Geometry check sheet. Reference: the model listing, model coordinates, mm. Face numbers are marked on the shaded views. A direction names the side the tool comes from. Give positions to 0.01 mm unless a question says otherwise; leave off trailing zeros. Write each loop counter-clockwise with the first axis right and the second up, starting at its lowest first coordinate (ties: lowest second). Pieces come first, ordered by that corner, then holes.
(1) Cross-section at A-A (z = -4). Record the boundary of the cut face in (x, y) (3 decimals).
(2) Mould release check, pull along X, two halves, no side actions. Record for the marked faces 6, 7 and 8: +X half, -X half, draft (parallel to the pull), parting line (faces both ways), or undercut.
(3) Tool access check on the marked faces 1, 2, 3, 4 and 5. Record the directions out of +Z, -Z, +X, -X, +Y, -Y that give a thin tool (end or side, any length) a straight path to the whole face; none if there is none.
(4) Thickness scan on line 1 along Z through (x, y) = (38, -43) (3 decimals); line 2 along Y through (x, z) = (-9.5, 23.5); line 3 along Z through (x, y) = (104.5, -12) (3 decimals). Record the ranges inside material, lowest first.
(5) Depth check by flat-ended pin: P1, Ø15.5, axis at x = 21, z = 35, coming from the -Y side; P2, Ø3, axis at x = 33.5, y = -19.5, coming from the +Z side; P3, Ø3, axis at y = -1, z = 18.5, coming from the +X side (3 decimals). Enter the tip coordinate at first touch or a pass-through.
(6) Cross-section at B-B (y = 47.5). Record the boundary of the cut face in (x, z) (3 decimals), and give its area (3 significant figures).
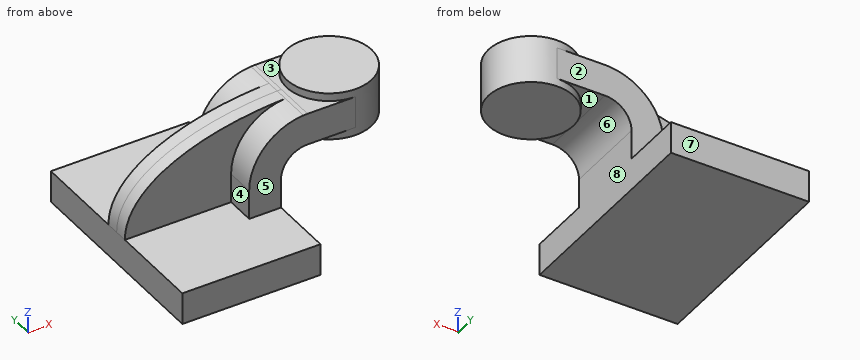
```python
from build123d import *

# Parameters (mm, degrees)
F1_DEPTH = 63.5
F0_W     = 25.4
F0_H     = 19.05
F2_DEPTH = 25.4
F3_DEPTH = 7.9375


with BuildPart() as f1:
    # F0 (on Front) → F1 (new body, symmetric)
    with BuildSketch(Plane.XZ):
        Polygon((41.275, -9.525), (41.275, 9.525), (22.225, 9.525), (-41.275, 9.525), (-41.275, -9.525), align=None)
    extrude(amount=F1_DEPTH, both=True)

    # F0 (on Front) → F2 (join, symmetric)
    with BuildSketch(Plane.XZ):
        with BuildLine():
            Line((22.225, 9.525), (41.275, 9.525))
            Line((41.275, 9.525), (41.275, 27.0002))
            ThreePointArc((41.275, 27.0002), (45.9246798487, 38.2255201513), (57.15, 42.8752))
            Line((57.15, 42.8752), (60.325, 42.8752))
            Line((60.325, 42.8752), (60.325, 61.9252))
            Line((60.325, 61.9252), (57.15, 61.9252))
            add(Edge.make_bspline(
                [(54.6808253359, 61.8378061387), (55.500532419, 61.870850227), (56.3236165266, 61.8999908241), (57.15, 61.9252)],
                knots=[109.8921913534, 109.8921913534, 109.8921913534, 109.8921913534, 111.5045361635, 111.5045361635, 111.5045361635, 111.5045361635], degree=3))
            ThreePointArc((54.6808253359, 61.8378061387), (31.5962179889, 50.806918588), (22.225, 27.0002))
            Line((22.225, 27.0002), (22.225, 9.525))
        make_face()
        with Locations((73.025, 52.4002)):
            Rectangle(F0_W, F0_H)
    extrude(amount=F2_DEPTH, both=True)

    # F0 (on Front) → F3 (join, symmetric)
    with BuildSketch(Plane.XZ):
        with BuildLine():
            Line((-41.275, 9.525), (22.225, 9.525))
            Line((22.225, 9.525), (22.225, 27.0002))
            ThreePointArc((22.225, 27.0002), (31.5962179889, 50.806918588), (54.6808253359, 61.8378061387))
            add(Edge.make_bspline(
                [(-41.275, 9.525), (-41.3688876605, 39.2003932287), (-1.1877500898, 59.5856282852), (54.6808253359, 61.8378061387)],
                knots=[0, 0, 0, 0, 109.8921913534, 109.8921913534, 109.8921913534, 109.8921913534], degree=3))
        make_face()
    extrude(amount=F3_DEPTH, both=True)

    # F0 (on Front) → F4 (revolve)
    with BuildSketch(Plane.XZ):
        Polygon((85.725, 61.9252), (85.725, 42.8752), (85.725, 38.1), (111.125, 38.1), (111.125, 66.675), (85.725, 66.675), align=None)
    revolve(axis=Axis((85.725, 0, 52.3875), (0, 0, -1)))


solid = f1.part
```
Reply:
1. outline: (-41.275, -63.5) - (41.275, -63.5) - (41.275, 63.5) - (-41.275, 63.5) - close
2. face 6: undercut
2. face 7: draft
2. face 8: +X half
3. face 1: -Z
3. face 2: +Z, +X, -X, +Y
3. face 3: +Z, -X
3. face 4: +Z, -X, -Y
3. face 5: +Z, +X, -X, -Y
4. line 1: z = -9.525 to 9.525
4. line 2: y = -7.94 to 7.94
4. line 3: z = 38.1 to 66.675
5. P1: stops at y = -25.4
5. P2: stops at z = 54
5. P3: stops at x = 41.275
6. outline: (-41.275, -9.525) - (41.275, -9.525) - (41.275, 9.525) - (-41.275, 9.525) - close
6. area: 1,570 mm2
